from build123d import *

# Parameters (mm, degrees)
SKETCH_1_R          = 15
EXTRUDE_1_DEPTH     = 8
SKETCH_2_R          = 17
SKETCH_2_R_2        = 15
EXTRUDE_2_DEPTH     = 1
SKETCH_3_R          = 1.5
CUT_EXTRUDE_1_DEPTH = 26.337718919
EXTRUDE_START       = -1
SKETCH_4_R          = 17
SKETCH_4_R_2        = 15
EXTRUDE_3_DEPTH     = 1
SKETCH_5_R          = 17
EXTRUDE_4_DEPTH     = 3
SKETCH_6_R          = 1.5
CUT_EXTRUDE_6_DEPTH = 1


with BuildPart() as part:
    # 草图1 → 凸台-拉伸1 (new body)
    with BuildSketch(Plane.XY):
        Circle(SKETCH_1_R)
    extrude(amount=EXTRUDE_1_DEPTH)

    # 草图2 → 凸台-拉伸2 (add)
    with BuildSketch(Plane(origin=(0, 0, 0), x_dir=(-1, 0, 0), z_dir=(0, 0, -1))):
        Circle(SKETCH_2_R)
        Circle(SKETCH_2_R_2, mode=Mode.SUBTRACT)
    extrude(amount=-EXTRUDE_2_DEPTH)

    # 草图3 → 切除-拉伸1 (cut, through all)
    with BuildSketch(Plane.XY.offset(8)):
        with Locations((0, 11)):
            Circle(SKETCH_3_R)
        with Locations((9.526279442, 5.5)):
            Circle(SKETCH_3_R)
        with Locations((9.526279442, -5.5)):
            Circle(SKETCH_3_R)
        with Locations((0, -11)):
            Circle(SKETCH_3_R)
        with Locations((-9.526279442, -5.5)):
            Circle(SKETCH_3_R)
        with Locations((-9.526279442, 5.5)):
            Circle(SKETCH_3_R)
    extrude(amount=-CUT_EXTRUDE_1_DEPTH, mode=Mode.SUBTRACT)

    # 草图4 → 凸台-拉伸3 (add)
    with BuildSketch(Plane.XY.offset(8).offset(EXTRUDE_START)):
        with Locations(Location((0, 0, 0), (0, 0, 180))):
            Circle(SKETCH_4_R)
        with Locations(Location((0, 0, 0), (0, 0, 180))):
            Circle(SKETCH_4_R_2, mode=Mode.SUBTRACT)
    extrude(amount=EXTRUDE_3_DEPTH)

    # 草图5 → 凸台-拉伸4 (add)
    with BuildSketch(Plane.XY.offset(8)):
        with Locations(Location((0, 0, 0), (0, 0, 180))):
            Circle(SKETCH_5_R)
    extrude(amount=EXTRUDE_4_DEPTH)

    # 草图6 → 切除-拉伸6 (cut)
    with BuildSketch(Plane.XY.offset(11)):
        with Locations((0, 11)):
            Circle(SKETCH_6_R)
        with Locations((9.526279442, 5.5)):
            Circle(SKETCH_6_R)
        with Locations((9.526279442, -5.5)):
            Circle(SKETCH_6_R)
        with Locations((0, -11)):
            Circle(SKETCH_6_R)
        with Locations((-9.526279442, -5.5)):
            Circle(SKETCH_6_R)
        with Locations((-9.526279442, 5.5)):
            Circle(SKETCH_6_R)
    extrude(amount=-CUT_EXTRUDE_6_DEPTH, mode=Mode.SUBTRACT)


solid = part.part
The listing builds one solid part. Answer for the finished solid, in the listing's coordinates (mm). A direction names the side the tool comes from. Give positions to 0.01 mm unless a question says otherwise; leave off trailing zeros. Loops run counter-clockwise (first coordinate to the right, second up) from the corner with the lowest first, then second, coordinate; pieces in that order, holes last. Notation, with made-up numbers: (52.5, 42) - (99.5, 42) arc R20 ccw to (99.5, 52) - close; hole circle Ø11 at (-31.75, 83.25). An arc over 180 degrees is marked (long way). Use one line per item in the form item = value.
1. Given pin 1 Ø2.5 at (x, y) = (9.53, -5.5) entering from -Z; pin 2 Ø1 at (x, z) = (9.5, 10) entering from +Y; pin 3 Ø1.5 at (y, z) = (-1, 1.5) entering from +X, each flat-ended and moving along its own axis, determine where each tip first touches the part or whether it passes through.
Calculated:
pin_1 = 8
pin_2 = 14.42
pin_3 = 16.99
2. Which of the six approach directions +Z, -Z, +X, -X, +Y, -Y give full straight-line access (tool end or side, diameter ignored) to faces 1 (the face through (-10, 6, 10)), 2 (the face through (2.213, -16.855, 8.972)), 3 (the face through (-11.025, -5.434, 4.056))?
Calculated:
face_1 = +Z
face_2 = +Z, -Z
face_3 = -Z
3. Section A-A on y = 0 is taken. Give the vertices of the cut face in (x, z).
Calculated:
outline = (-17, 0) - (17, 0) - (17, 1) - (15, 1) - (15, 7) - (17, 7) - (17, 11) - (-17, 11) - (-17, 7) - (-15, 7) - (-15, 1) - (-17, 1) - close
4. Section B-B on z = 2 is taken. Give the vertices of the cut face in (x, y).
Calculated:
outline = circle Ø30 at (0, 0); hole circle Ø3 at (-9.53, -5.5); hole circle Ø3 at (-9.53, 5.5); hole circle Ø3 at (0, -11); hole circle Ø3 at (0, 11); hole circle Ø3 at (9.53, -5.5); hole circle Ø3 at (9.53, 5.5)
5. Section D-D on z = 8.75 is taken. Give the vertices of the cut face in (x, y).
Calculated:
outline = circle Ø34 at (0, 0)
6. Find the intervals of material crossed by line 1 along Z through (x, y) = (4, -14.5); line 2 along Y through (x, z) = (-1, 3.5); line 3 along Y through (x, z) = (-8.5, 5.5), in increasing order. Write a range as [from, to].
Calculated:
line_1 = [0, 1], [7, 11]
line_2 = [-14.97, -12.12], [-9.88, 9.88], [12.12, 14.97]
line_3 = [-12.36, -6.59], [-4.41, 4.41], [6.59, 12.36]
7. The mould has two halves that part along Z. Classify faces 4 (the face through (-14.985, 0.66, 3.958)), 5 (the face through (10.9, 4.9, 10.5)), 6 (the face through (0, -11, 8)), 7 (the face through (-6, -14, 1)): pulls with the +Z half, pulls with the -Z half, needs draft (parallel to the pull), parting line crosses it, or undercut.
Calculated:
face_4 = undercut
face_5 = needs draft
face_6 = pulls with the -Z half
face_7 = undercut
8. Section C-C on x = 0 is taken. Give the vertices of the cut face in (y, z).
Calculated:
outline = (-17, 0) - (-12.5, 0) - (-12.5, 8) - (-9.5, 8) - (-9.5, 0) - (9.5, 0) - (9.5, 8) - (12.5, 8) - (12.5, 0) - (17, 0) - (17, 1) - (15, 1) - (15, 7) - (17, 7) - (17, 11) - (12.5, 11) - (12.5, 10) - (9.5, 10) - (9.5, 11) - (-9.5, 11) - (-9.5, 10) - (-12.5, 10) - (-12.5, 11) - (-17, 11) - (-17, 7) - (-15, 7) - (-15, 1) - (-17, 1) - close
